Geometry: final body of the model. Coordinates: model frame, mm. Give positions to 0.01 mm unless a question says otherwise; leave off trailing zeros. Write each loop counter-clockwise with the first axis right and the second up, starting at its lowest first coordinate (ties: lowest second). Pieces come first, ordered by that corner, then holes. Notation, with made-up numbers: (79, 47) - (99, 47) arc R25 cw to (99, 63) - close; hole circle Ø6 at (25.25, -31.75). An arc over 180 degrees is marked (long way). Return JSON: item names as keys, results as strings.
from build123d import *

# Parameters (mm, degrees)
SKETCH1_W           = 88
SKETCH1_H           = 70
BOSS_EXTRUDE1_DEPTH = 5
SKETCH2_R           = 1.375
CUT_EXTRUDE1_DEPTH  = 5
CUT_EXTRUDE2_START  = -5
SKETCH4_R           = 1.375
CUT_EXTRUDE2_DEPTH  = 5
SKETCH5_R           = 15
CUT_EXTRUDE3_DEPTH  = 57.444663167


with BuildPart() as part:
    # Sketch1 → Boss-Extrude1 (new body)
    with BuildSketch(Plane(origin=(0, 0, 0), x_dir=(1, 0, 0), z_dir=(0, 1, 0))):
        Rectangle(SKETCH1_W, SKETCH1_H)
    extrude(amount=BOSS_EXTRUDE1_DEPTH)

    # Sketch2 → Cut-Extrude1 (cut)
    with BuildSketch(Plane.XY.offset(35)):
        with Locations((-10.55, 2.5)):
            Circle(SKETCH2_R)
        with Locations((29.45, 2.5)):
            Circle(SKETCH2_R)
    extrude(amount=-CUT_EXTRUDE1_DEPTH, mode=Mode.SUBTRACT)

    # Sketch4 → Cut-Extrude2 (cut)
    with BuildSketch(Plane(origin=(0, 0, -35), x_dir=(-1, 0, 0), z_dir=(0, 0, -1)).offset(CUT_EXTRUDE2_START)):
        with Locations(Location((-29.45, 2.5, 0), (0, 0, 180))):
            Circle(SKETCH4_R)
        with Locations(Location((10.55, 2.5, 0), (0, 0, 180))):
            Circle(SKETCH4_R)
    extrude(amount=CUT_EXTRUDE2_DEPTH, mode=Mode.SUBTRACT)

    # Sketch5 → Cut-Extrude3 (cut, through all)
    with BuildSketch(Plane(origin=(0, 5, 0), x_dir=(1, 0, 0), z_dir=(0, 1, 0))):
        with Locations(Location((-18.469657797, -10, 0), (0, 0, 270))):
            Circle(SKETCH5_R)
    extrude(amount=-CUT_EXTRUDE3_DEPTH, mode=Mode.SUBTRACT)


solid = part.part
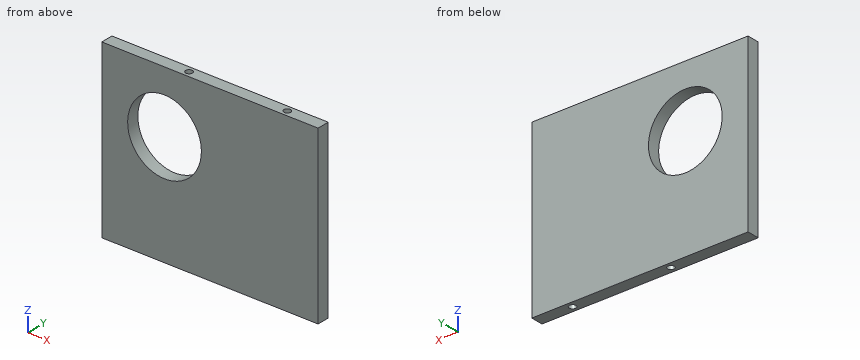
Q1. Section query A-A, the plane z = 15.5. Return the cut outline in (x, y), plus the area to 3 significant figures.
Answer key:
{"outline": "(-44, 0) - (-32.42, 0) - (-32.42, 5) - (-44, 5) - close; (-4.51, 0) - (44, 0) - (44, 5) - (-4.51, 5) - close", "area": "300 mm^2"}
Q2. Material intervals for probe 1 along X at (y, z) = (2.5, -31.6) (3 decimals); probe 2 along Y at (x, z) = (29.45, -33.75) (3 decimals); probe 3 along Z at (x, y) = (29, 3.35), sorted ascending. Write a range as [from, to].
Answer key:
{"probe 1": "x = [-44, -11.925], [-9.175, 28.075], [30.825, 44]", "probe 2": "y = [0, 1.125], [3.875, 5]", "probe 3": "z = [-30, 30]"}
Q3. Section query C-C, the plane y = 2.5. Return the cut outline in (x, z) (3 decimals), plus the area to 3 significant figures.
Answer key:
{"outline": "(-44, -35) - (-11.925, -35) - (-11.925, -30) - (-9.175, -30) - (-9.175, -35) - (28.075, -35) - (28.075, -30) - (30.825, -30) - (30.825, -35) - (44, -35) - (44, 35) - (30.825, 35) - (30.825, 30) - (28.075, 30) - (28.075, 35) - (-9.175, 35) - (-9.175, 30) - (-11.925, 30) - (-11.925, 35) - (-44, 35) - close; hole circle Ø30 at (-18.47, 10)", "area": "5,400 mm^2"}
Q4. Pin query (flat end, axial travel): P1, Ø0.8, axis at x = -11, y = 3, coming from the +Z side; P2, Ø3, axis at x = 29.45, y = 2.5, coming from the -Z side; P3, Ø1.6, axis at x = -10.55, y = 2.5, coming from the -Z side. Return the tip coordinate at first contact, or that it passes through.
Answer key:
{"P1": "stops at z = 30", "P2": "stops at z = -35", "P3": "stops at z = -30"}
Q5. Section query B-B, the plane x = -10.55. Return the cut outline in (y, z) (3 decimals).
Answer key:
{"outline": "(0, -35) - (1.125, -35) - (1.125, -30) - (3.875, -30) - (3.875, -35) - (5, -35) - (5, -2.739) - (0, -2.739) - close; (0, 22.739) - (5, 22.739) - (5, 35) - (3.875, 35) - (3.875, 30) - (1.125, 30) - (1.125, 35) - (0, 35) - close"}
Q6. Section query D-D, the plane x = 29.45. Return the cut outline in (y, z) (3 decimals), plus the area to 4 significant figures.
Answer key:
{"outline": "(0, -35) - (1.125, -35) - (1.125, -30) - (3.875, -30) - (3.875, -35) - (5, -35) - (5, 35) - (3.875, 35) - (3.875, 30) - (1.125, 30) - (1.125, 35) - (0, 35) - close", "area": "322.5 mm^2"}
